Work out the finished part from the listing and answer in its coordinate system (mm). Face numbers are marked on the shaded views. A direction names the side the tool comes from. Round coordinates to 2 decimals unless told otherwise and drop trailing zeros. Loops run counter-clockwise (first coordinate to the right, second up) from the corner with the lowest first, then second, coordinate; pieces in that order, holes last. Notation, with made-up numbers: M 80.5,89.25 L 91.5,89.25 A11 cw 91.5,98.25 Z; hole C 32,-36.75 d6. An arc over 180 degrees is marked long. One line per item, written item: value.
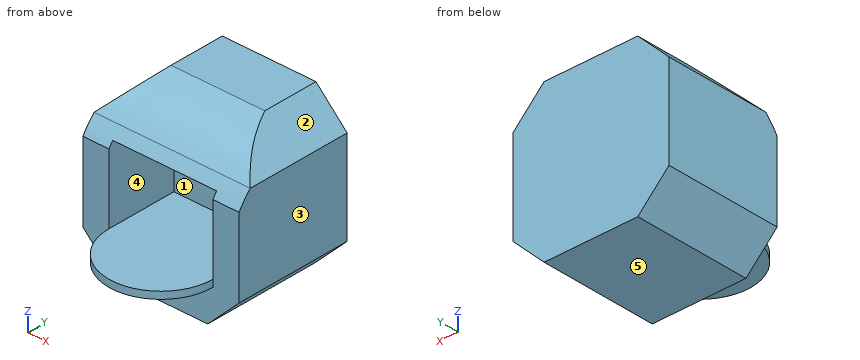
```python
from build123d import *

# Parameters (mm, degrees)
F0_W     = 200
F0_H     = 200
F1_DEPTH = 75
F2_SIZE  = 40
F3_W     = 133.0324709415
F3_H     = 95.5820605159
F4_DEPTH = 90
F6_DEPTH = 200.9
F8_DEPTH = 9


with BuildPart() as f1:
    # F0 (on Front) → F1 (new body, symmetric)
    with BuildSketch(Plane.XZ):
        Rectangle(F0_W, F0_H)
    extrude(amount=F1_DEPTH, both=True)

    # F2
    f2_edges = [f1.edges().sort_by_distance(p)[0] for p in [
        (100, 0, 100),
        (-100, 0, 100),
        (-100, 0, -100),
        (100, 0, -100),
    ]]
    chamfer(f2_edges, length=F2_SIZE)

    # F3 (on face) → F4 (cut)
    with BuildSketch(Plane.XZ.offset(75)):
        Rectangle(F3_W, F3_H)
    extrude(amount=-F4_DEPTH, mode=Mode.SUBTRACT)

    # F5 (on face) → F6 (cut)
    with BuildSketch(Plane.YZ.offset(100)):
        with BuildLine():
            Line((-95.2423661947, -20.9655482322), (-87.9932567477, -22.9425765574))
            add(Edge.make_bspline(
                [(-87.9932567477, -22.9425765574), (-88.9180534775, -7.4435947272), (-90.1399220102, 13.0341141319), (-78.4659039791, 35.1732019961), (-75, 40.5114376133)],
                knots=[0, 0, 0, 0, 0.2716788235, 0.3589500209, 0.3589500209, 0.3589500209, 0.3589500209], degree=3))
            Line((-75, 40.5114376133), (-75, 60))
            Line((-75, 60), (-59.3654634192, 60))
            add(Edge.make_bspline(
                [(-59.3654634192, 60), (-50.780700635, 68.9119189144), (-16.3848726556, 97.0242933868), (26.186759324, 107.4256565423), (56.3297905028, 114.7903874516)],
                knots=[0.4677889294, 0.4677889294, 0.4677889294, 0.4677889294, 0.6231656117, 1, 1, 1, 1], degree=3))
            Line((56.3297905028, 114.7903874516), (-23.4103426337, 159.6030145884))
            Line((-23.4103426337, 159.6030145884), (-86.6752415895, 159.6030145884))
            Line((-86.6752415895, 159.6030145884), (-134.7829252481, 0))
            Line((-134.7829252481, 0), (-95.2423661947, -20.9655482322))
        make_face()
        with BuildLine():
            Line((-75, 60), (-75, 40.5114376133))
            add(Edge.make_bspline(
                [(-75, 40.5114376133), (-70.6775520716, 47.1689346541), (-65.3789539733, 53.7573417509), (-59.3654634192, 60)],
                knots=[0.3589500209, 0.3589500209, 0.3589500209, 0.3589500209, 0.4677889294, 0.4677889294, 0.4677889294, 0.4677889294], degree=3))
            Line((-59.3654634192, 60), (-75, 60))
        make_face()
    extrude(amount=-F6_DEPTH, mode=Mode.SUBTRACT)

    # F7 (on face) → F8 (join)
    with BuildSketch(Plane.XY.offset(-47.7910302579)):
        with BuildLine():
            Line((66.5162354708, -75), (-66.5162354708, -75))
            ThreePointArc((-66.5162354708, -75), (0, -141.5162354708), (66.5162354708, -75))
        make_face()
    extrude(amount=-F8_DEPTH)


solid = f1.part
```
1) The mould has two halves that part along Z. Classify the marked faces 3, 4 and 5: +Z half, -Z half, draft (parallel to the pull), parting line (faces both ways), or undercut.
Check values:
face 3: draft
face 4: undercut
face 5: -Z half
2) Find section D-D (y = -87). Give the vertices of the cut face in (x, z), then the cut area to 3 significant figures.
Check values:
outline: M -65.42,-56.79 L 65.42,-56.79 L 65.42,-47.79 L -65.42,-47.79 Z
area: 1,180 mm2
3) Find the intervals of material crossed by probe 1 along X at (y, z) = (-56.5, 15); probe 2 along Y at (x, z) = (-83.5, -35), in increasing order. Write a range as from..to.
Check values:
probe 1: -100..-66.52, 66.52..100
probe 2: -75..75
4) Find section A-A (z = -4). Give the vertices of the cut face in (x, y), then the cut area to 3 significant figures.
Check values:
outline: M -100,-75 L -66.52,-75 L -66.52,15 L 66.52,15 L 66.52,-75 L 100,-75 L 100,75 L -100,75 Z
area: 18,000 mm2
5) For the marked faces 1 and 2, determine the directions among +Z, -Z, +X, -X, +Y, -Y from which every point of the face is accessible in a straight line to the end or side of a thin tool.
Check values:
face 1: -Y
face 2: +Z, +X, +Y, -Y
6) Find section B-B (y = 19.5). Give the vertices of the cut face in (x, z).
Check values:
outline: M -100,-60 L -60,-100 L 60,-100 L 100,-60 L 100,60 L 60,100 L -60,100 L -100,60 Z
7) Find section C-C (y = -122.5). Give the vertices of the cut face in (x, z), then the cut area to 3 significant figures.
Check values:
outline: M -46.56,-56.79 L 46.56,-56.79 L 46.56,-47.79 L -46.56,-47.79 Z
area: 838 mm2
8) Each of these flat-tipped pins is pushed along its axis until it touches: pin 1 (2 mm diameter, centred on x = 74, y = -66.5, fed in from +Z); pin 2 (4 mm diameter, centred on x = 38, y = -103, fed in from -Z); pin 3 (2 mm diameter, centred on x = 26.5, y = -46, fed in from +Z). Where does it stop, or does it pass through?
Check values:
pin 1: z = 53.22
pin 2: z = -56.79
pin 3: z = 73.14
